from build123d import *

# Parameters (mm, degrees)
SKETCH008_W     = 54
SKETCH008_H     = 19
PAD006_DEPTH    = 2.5
SKETCH009_R     = 2.5
POCKET002_DEPTH = 2.501
FILLET007_R     = 2
FILLET008_R     = 2
FILLET009_R     = 2
FILLET010_R     = 2
PAD007_DEPTH    = 0.5


with BuildPart() as part:
    # Sketch008 → Pad006 (new body)
    with BuildSketch(Plane.XY):
        Rectangle(SKETCH008_W, SKETCH008_H)
    extrude(amount=PAD006_DEPTH)

    # Sketch009 (on Face6 of Pad006) → Pocket002 (cut, through all)
    with BuildSketch(Plane.XY.offset(2.5)):
        with Locations((-24, 5)):
            Circle(SKETCH009_R)
        with Locations((24, 5)):
            Circle(SKETCH009_R)
        with Locations((24, -5)):
            Circle(SKETCH009_R)
        with Locations((-24, -5)):
            Circle(SKETCH009_R)
    extrude(amount=-POCKET002_DEPTH, mode=Mode.SUBTRACT)

    # Fillet007
    fillet007_edges = [part.edges().sort_by_distance(p)[0] for p in [
        (27, 9.5, 1.25),
    ]]
    fillet(fillet007_edges, radius=FILLET007_R)

    # Fillet008
    fillet008_edges = [part.edges().sort_by_distance(p)[0] for p in [
        (-27, 9.5, 1.25),
    ]]
    fillet(fillet008_edges, radius=FILLET008_R)

    # Fillet009
    fillet009_edges = [part.edges().sort_by_distance(p)[0] for p in [
        (-27, -9.5, 1.25),
    ]]
    fillet(fillet009_edges, radius=FILLET009_R)

    # Fillet010
    fillet010_edges = [part.edges().sort_by_distance(p)[0] for p in [
        (27, -9.5, 1.25),
    ]]
    fillet(fillet010_edges, radius=FILLET010_R)

    # Sketch010 → Pad007 (join, symmetric)
    with BuildSketch(Plane.XZ):
        Polygon((-27, 0), (-19.6, 0), (-19.6, -2), align=None)
    pad007 = extrude(amount=PAD007_DEPTH, both=True)

    # Mirrored: Pad007 across Sketch010 V_Axis
    add(pad007.mirror(Plane(origin=(0, 0, 0), x_dir=(0, -1, 0), z_dir=(1, 0, 0))))


solid = part.part
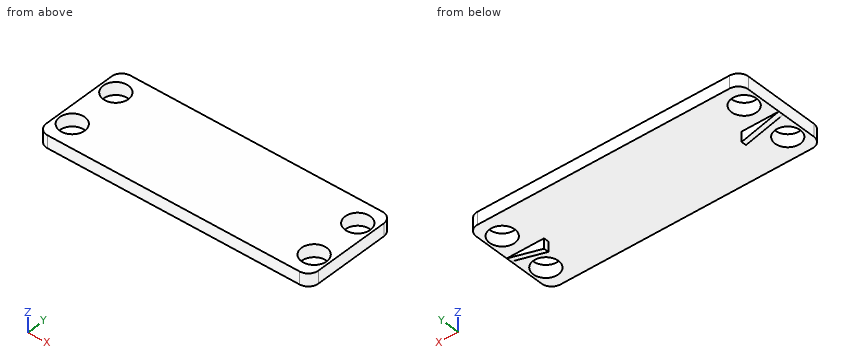
Geometry: final body of the model. Coordinates: model frame, mm. Coordinates: 2 decimals unless noted, no trailing zeros. Loops run counter-clockwise (first coordinate to the right, second up) from the corner with the lowest first, then second, coordinate; pieces in that order, holes last. Notation, with made-up numbers: (48, 80) - (104, 80) arc R14 ccw to (104, 86) - close; hole circle Ø4 at (37, 63.25). An arc over 180 degrees is marked (long way). One line per question, with ' | ' between items. Start each with the question number.
(1) Cut plane B-B on z = -1.3. Output: boundary loops of the cut face in (x, y), and give its area (3 significant figures).
(2) First-contact query: pin 1 (4 mm diameter, centred on x = 24, y = -5, fed in from +Z); pin 2 (6.5 mm diameter, centred on x = -24, y = 5, fed in from +Z); pin 3 (1.6 mm diameter, centred on x = 22.5, z = -1.5, fed in from +Y); pin 4 (1.5 mm diameter, centred on x = 4.5, y = 2, fed in from -Z). Flat tips, straight axial feed; report the tip coordinate or a pass-through.
(3) Cut plane D-D on y = -5. Output: boundary loops of the cut face in (x, z).
(4) Cut plane C-C on x = 24. Output: boundary loops of the cut face in (y, z).
(5) Ray query, L1, parallel to Y at x = -24, z = 1.35; L2, parallel to Z at x = 24.5, y = -8.25; L3, parallel to X at y = -6, z = 0.45. Return the intervals inside material, ascending. Write a range as from..to.
(6) Cut plane A-A on y = 3.5. Output: boundary loops of the cut face in (x, z), and give its area (3 significant figures).
Here are the results:
1) outline: (-22.19, -0.5) - (-19.6, -0.5) - (-19.6, 0.5) - (-22.19, 0.5) - close; (19.6, -0.5) - (22.19, -0.5) - (22.19, 0.5) - (19.6, 0.5) - close | area: 5.18 mm²
2) pin 1: through | pin 2: z = 2.5 | pin 3: y = 0.5 | pin 4: z = 0
3) outline: (-27, 0) - (-26.5, 0) - (-26.5, 2.5) - (-27, 2.5) - close; (-21.5, 0) - (21.5, 0) - (21.5, 2.5) - (-21.5, 2.5) - close; (26.5, 0) - (27, 0) - (27, 2.5) - (26.5, 2.5) - close
4) outline: (-9.5, 0) - (-7.5, 0) - (-7.5, 2.5) - (-9.5, 2.5) - close; (-2.5, 0) - (-0.5, 0) - (-0.5, -0.81) - (0.5, -0.81) - (0.5, 0) - (2.5, 0) - (2.5, 2.5) - (-2.5, 2.5) - close; (7.5, 0) - (9.5, 0) - (9.5, 2.5) - (7.5, 2.5) - close
5) L1: -9.5..-7.5, -2.5..2.5, 7.5..9.5 | L2: 0..2.5 | L3: -27..-26.29, -21.71..21.71, 26.29..27
6) outline: (-27, 0) - (-26, 0) - (-26, 2.5) - (-27, 2.5) - close; (-22, 0) - (22, 0) - (22, 2.5) - (-22, 2.5) - close; (26, 0) - (27, 0) - (27, 2.5) - (26, 2.5) - close | area: 115 mm²
